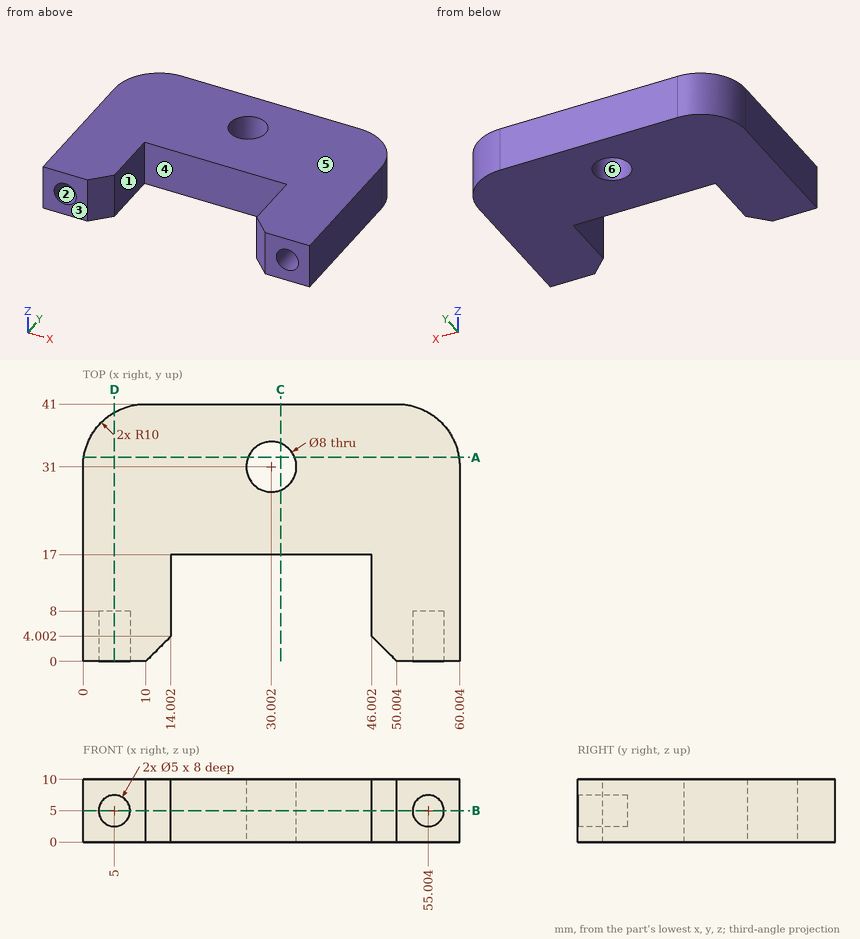
Verification items for this drawing (mm, ordinates from the low corner). A direction names the side the tool comes from. Coordinates: 2 decimals unless noted, no trailing zeros. Order: outer loops, then holes, each group sorted by start corner. A loop starts at its lowest first (then second) coordinate and runs counter-clockwise, first axis right, second up. Notation, with made-up numbers: M 33,38 L 59,38 A21 cw 59,44 Z; hole C -2,20.25 d1. An arc over 180 degrees is marked long. One line per item, written item: value. Start each with the question number.
Item 1: Sectioned sample at D-D on x = 5. Record the cut outline in (y, z).
Item 2: Mould release check, pull along Y, two halves, no side actions. Record for the marked faces 4, 5 and 6: pulls with the +Y half, pulls with the -Y half, needs draft (parallel to the pull), parting line crosses it, or undercut.
Item 3: Thickness scan on probe 1 along X at (y, z) = (5.25, 5) (1 decimal); probe 2 along X at (y, z) = (11.5, 4) (1 decimal); probe 3 along X at (y, z) = (1.5, 5) (1 decimal). Record the ranges inside material, lowest first.
Item 4: Sectioned sample at C-C on x = 31.5. Record the cut outline in (y, z), then the cut area to 3 significant figures.
Item 5: Sectioned sample at A-A on y = 32.5. Record the cut outline in (x, z) (1 decimal).
Item 6: Depth check by flat-ended pin: P1, Ø1.5, axis at x = 56, z = 6, coming from the -Y side; P2, Ø1, axis at x = 19.5, z = 4, coming from the -Y side. Enter the tip coordinate at first touch or a pass-through.
Item 7: Access from +Z, -Z, +X, -X, +Y, -Y to the whole of each face (thin tool, end or side, straight path). Record for the marked faces 1, 2 and 3.
Item 8: Sectioned sample at B-B on z = 5. Record the cut outline in (x, y) (1 decimal), then the cut area to 3 significant figures.
Calculated:
1. outline: M 0,0 L 39.66,0 L 39.66,10 L 0,10 L 0,7.5 L 8,7.5 L 8,2.5 L 0,2.5 Z
2. face 4: pulls with the -Y half
2. face 5: needs draft
2. face 6: undercut
3. probe 1: 0 to 2.5, 7.5 to 14, 46 to 52.5, 57.5 to 60
3. probe 2: 0 to 14, 46 to 60
3. probe 3: 0 to 2.5, 7.5 to 11.5, 48.5 to 52.5, 57.5 to 60
4. outline: M 17,0 L 27.29,0 L 27.29,10 L 17,10 Z; M 34.71,0 L 41,0 L 41,10 L 34.71,10 Z
4. area: 166 mm^2
5. outline: M 0.1,0 L 26.3,0 L 26.3,10 L 0.1,10 Z; M 33.7,0 L 59.9,0 L 59.9,10 L 33.7,10 Z
6. P1: y = 8
6. P2: y = 17
7. face 1: +Z, -Z, -Y
7. face 2: -Y
7. face 3: +Z, -Z, +X, -X, -Y
8. outline: M 0,0 L 2.5,0 L 2.5,8 L 7.5,8 L 7.5,0 L 10,0 L 14,4 L 14,17 L 46,17 L 46,4 L 50,0 L 52.5,0 L 52.5,8 L 57.5,8 L 57.5,0 L 60,0 L 60,31 A10 ccw 50,41 L 10,41 A10 ccw 0,31 Z; hole C 30,31 d8
8. area: 1,730 mm^2
